Here's the drawing with two shaded views (mm, measured from the low corner). I have some questions. A direction names the side the tool comes from. Round coordinates to 2 decimals unless told otherwise and drop trailing zeros. Order: outer loops, then holes, each group sorted by start corner. A loop starts at its lowest first (then second) coordinate and runs counter-clockwise, first axis right, second up. Notation, with made-up numbers: (-30, -8.5) -> (-3, -8.5) arc R18 ccw to (-3, 11.5) -> close; hole circle Ø8 at (37.25, 21.25). An arc over 180 degrees is marked (long way). Answer in a Markdown table with one row per item.
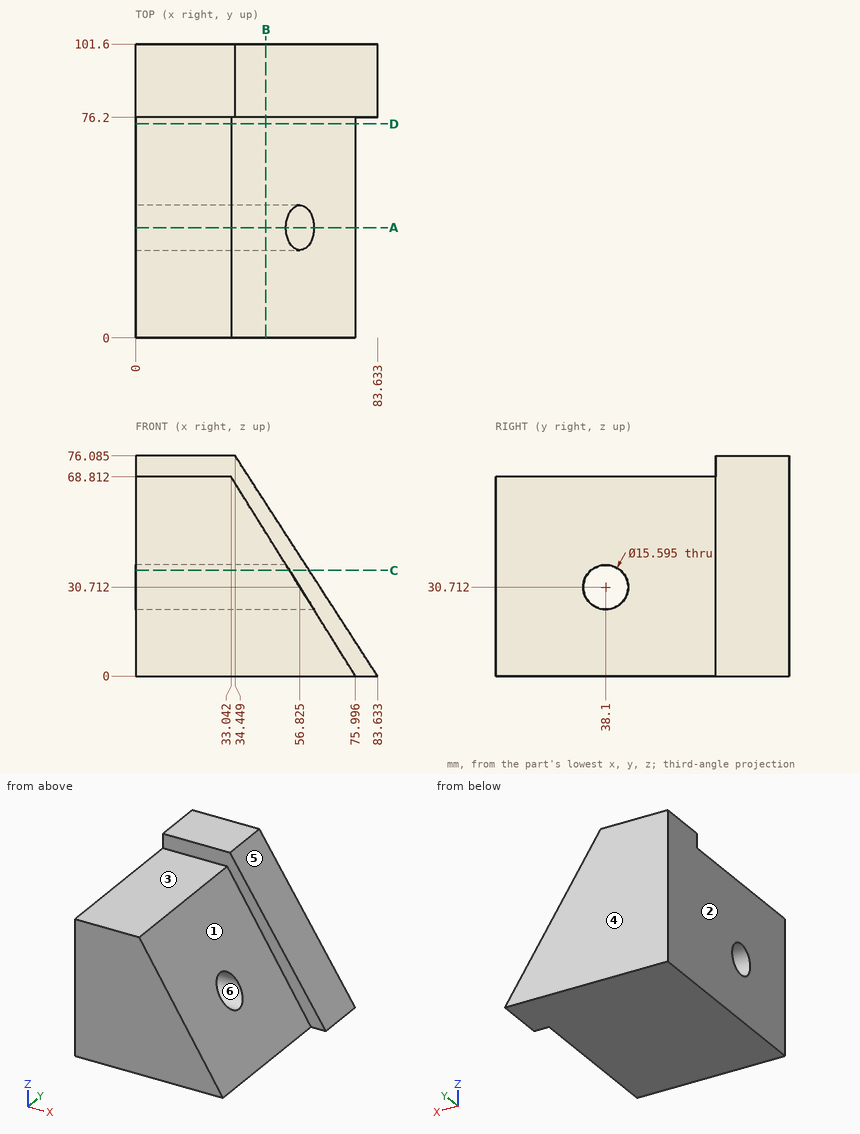
1. Suppose I cut it at C-C on z = 36.5. Write out the boundary of the cut face in (x, y) (1 decimal), then the cut area to 3 significant figures.
Numbers:
| item | result |
|---|---|
| outline | (0, 0) -> (53.2, 0) -> (53.2, 32.9) -> (0, 32.9) -> close; (0, 43.3) -> (53.2, 43.3) -> (53.2, 76.2) -> (60, 76.2) -> (60, 101.6) -> (0, 101.6) -> close |
| area | 5,020 mm2 |
2. Suppose I cut it at A-A on y = 38.1. Write out the boundary of the cut face in (x, z) (1 decimal), then the cut area to 3 significant figures.
Numbers:
| item | result |
|---|---|
| outline | (0, 0) -> (76, 0) -> (61.7, 22.9) -> (0, 22.9) -> close; (0, 38.5) -> (52, 38.5) -> (33, 68.8) -> (0, 68.8) -> close |
| area | 2,870 mm2 |
3. For pin 1 Ø2 at (y, z) = (76.5, 26.5) entering from +X; pin 2 Ø16.5 at (x, y) = (23.5, 36) entering from +Z, each with a flat end and sliding along its axis, tell me the tip position at first contact or that it passes through.
Numbers:
| item | result |
|---|---|
| pin 1 | stops at x = 67.15 |
| pin 2 | stops at z = 68.81 |
4. For the marked faces 1, 2 and 3, which set-ups out of +Z, -Z, +X, -X, +Y, -Y let a thin tool reach every point of the face, with its end or its side?
Numbers:
| item | result |
|---|---|
| face 1 | +Z, +X, -Y |
| face 2 | +Z, -Z, -X, +Y, -Y |
| face 3 | +Z, +X, -X, -Y |
5. Suppose I cut it at D-D on y = 74. Write out the boundary of the cut face in (x, z) (1 decimal), then the cut area to 3 significant figures.
Numbers:
| item | result |
|---|---|
| outline | (0, 0) -> (76, 0) -> (33, 68.8) -> (0, 68.8) -> close |
| area | 3,750 mm2 |
6. We'd pull the mould along Y, two halves only. Please class the marked faces 4, 5 and 6: released by +Y, released by -Y, zero draft, split by the parting line, or undercut.
Numbers:
| item | result |
|---|---|
| face 4 | released by +Y |
| face 5 | zero draft |
| face 6 | undercut |
7. Please list where these lines run through material, in increasing order: line 1 along Z through (x, y) = (15, 38) (1 decimal); line 2 along Z through (x, y) = (5, 55.5); line 3 along Z through (x, y) = (42, 38.1) (1 decimal).
Numbers:
| item | result |
|---|---|
| line 1 | z = 0 to 22.9, 38.5 to 68.8 |
| line 2 | z = 0 to 68.81 |
| line 3 | z = 0 to 22.9, 38.5 to 54.5 |
8. Suppose I cut it at B-B on x = 45. Write out the boundary of the cut face in (y, z) (1 decimal).
Numbers:
| item | result |
|---|---|
| outline | (0, 0) -> (101.6, 0) -> (101.6, 59.8) -> (76.2, 59.8) -> (76.2, 49.7) -> (0, 49.7) -> close; hole circle Ø15.6 at (38.1, 30.7) |
